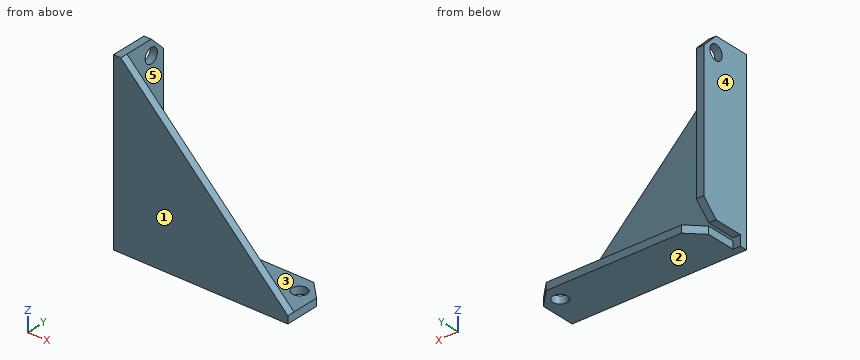
```python
from build123d import *

# Parameters (mm, degrees)
BOSS_EXTRUDE1_DEPTH = 3.175
SKETCH2_W           = 71.842048969
SKETCH2_H           = 3.175
BOSS_EXTRUDE2_DEPTH = 18.923
SKETCH3_W           = 3.175
SKETCH3_H           = 70.598963312
BOSS_EXTRUDE6_DEPTH = 18.923
CUT_EXTRUDE1_DEPTH  = 18.923
CUT_EXTRUDE2_DEPTH  = 18.923
SKETCH7_R           = 3.175
CUT_EXTRUDE3_DEPTH  = 18.923
SKETCH6_R           = 3.175
CUT_EXTRUDE4_DEPTH  = 18.923


with BuildPart() as part:
    # Sketch1 → Boss-Extrude1 (new body)
    with BuildSketch(Plane(origin=(0, 0, 0), x_dir=(1, 0, 0), z_dir=(0, 1, 0))):
        Polygon((-16.345355317, 62.119418011), (58.671693652, 62.119418011), (58.671693652, 58.944418011), (-13.170355317, -12.897630958), (-16.345355317, -12.897630958), align=None)
    extrude(amount=BOSS_EXTRUDE1_DEPTH)

    # Sketch2 → Boss-Extrude2 (add)
    with BuildSketch(Plane(origin=(0, 3.175, 0), x_dir=(1, 0, 0), z_dir=(0, 1, 0))):
        with Locations((22.750669167, 60.531918011)):
            Rectangle(SKETCH2_W, SKETCH2_H)
    extrude(amount=BOSS_EXTRUDE2_DEPTH)

    # Sketch3 → Boss-Extrude6 (add)
    with BuildSketch(Plane(origin=(0, 3.175, 0), x_dir=(1, 0, 0), z_dir=(0, 1, 0))):
        with Locations((-14.757855317, 22.401850698)):
            Rectangle(SKETCH3_W, SKETCH3_H)
    extrude(amount=BOSS_EXTRUDE6_DEPTH)

    # Sketch4 → Cut-Extrude1 (cut)
    with BuildSketch(Plane.ZY.offset(16.345355317)):
        Polygon((6.547630958, 22.098), (12.897630958, 15.748), (12.897630958, 22.098), align=None)
        Polygon((-57.701332354, 22.098), (-57.701332354, 15.748), (-51.351332354, 22.098), align=None)
    extrude(amount=-CUT_EXTRUDE1_DEPTH, mode=Mode.SUBTRACT)

    # Sketch5 → Cut-Extrude2 (cut)
    with BuildSketch(Plane(origin=(0, 0, -62.119418011), x_dir=(-1, 0, 0), z_dir=(0, 0, -1))):
        Polygon((13.170355317, 15.748), (6.820355317, 22.098), (13.170355317, 22.098), align=None)
        Polygon((-58.671693652, 14.834935127), (-51.408628779, 22.098), (-58.671693652, 22.098), align=None)
    extrude(amount=-CUT_EXTRUDE2_DEPTH, mode=Mode.SUBTRACT)

    # Sketch7 → Cut-Extrude3 (cut)
    with BuildSketch(Plane(origin=(-13.170355317, 0, 0), x_dir=(0, 0, -1), z_dir=(1, 0, 0))):
        with Locations((-6.547630958, 15.748)):
            Circle(SKETCH7_R)
    extrude(amount=-CUT_EXTRUDE3_DEPTH, mode=Mode.SUBTRACT)

    # Sketch6 → Cut-Extrude4 (cut)
    with BuildSketch(Plane.XY.offset(-58.944418011)):
        with Locations((51.408628779, 14.834935127)):
            Circle(SKETCH6_R)
    extrude(amount=-CUT_EXTRUDE4_DEPTH, mode=Mode.SUBTRACT)


solid = part.part
```
Could you check a few things on this model? Use its own coordinates, in mm. Face numbers are marked on the shaded views. A direction names the side the tool comes from. Round coordinates to 2 decimals unless told otherwise and drop trailing zeros. Loops run counter-clockwise (first coordinate to the right, second up) from the corner with the lowest first, then second, coordinate; pieces in that order, holes last. Notation, with made-up numbers: M -30,87 L -19,87 A20 cw -19,117 Z; hole C 22.25,-22 d1. An arc over 180 degrees is marked long. Write item = value, one per line.
1. Will these pins go through, and if not, where does the flat tip stop? P1, Ø5, axis at y = 15.75, z = 6.55, coming from the -X side; P2, Ø1, axis at y = 7.5, z = -60.5, coming from the -X side; P3, Ø2.5, axis at x = -14.5, y = 10, coming from the -Z side; P4, Ø10, axis at x = 5.5, y = 12.5, coming from the +Z side.
Results below:
P1 = through
P2 = -13.17
P3 = -57.7
P4 = -58.94
2. I want a section at C-C, the plane x = 14.5. Write out the boundary of the cut face in (y, z) (3 decimals), and give its area (3 significant figures).
Results below:
outline = M 0,-62.119 L 22.098,-62.119 L 22.098,-58.944 L 3.175,-58.944 L 3.175,-14.773 L 0,-14.773 Z
area = 210 mm²
3. I want a section at D-D, the plane z = -30.5. Write out the boundary of the cut face in (x, y) (3 decimals), and give its area (3 significant figures).
Results below:
outline = M -16.345,0 L 30.227,0 L 30.227,3.175 L -13.17,3.175 L -13.17,22.098 L -16.345,22.098 Z
area = 208 mm²
4. Which directions (+Z, -Z, +X, -X, +Y, -Y) give clear straight access to the entire face, cutting with the end or side of a thin tool? Please do the marked faces 3, 4 and 5.
Results below:
face_3 = +Z, +X, -X, +Y
face_4 = +Z, -Z, -X, +Y, -Y
face_5 = +Z, +X, +Y
5. I need wall thicknesses on probe 1 along Z at (x, y) = (53, 20.25); probe 2 along Y at (x, z) = (-12, -15) (3 decimals); probe 3 along X at (y, z) = (4.5, -6). Which ranges of each line are inside material? Lowest first, please.
Results below:
probe_1 = -62.12 to -58.94
probe_2 = 0 to 3.175
probe_3 = -16.35 to -13.17
6. I want a section at A-A, the plane y = 8. Write out the boundary of the cut face in (x, z), and give its area (3 significant figures).
Results below:
outline = M -16.35,-57.7 L -13.17,-57.7 L -13.17,12.9 L -16.35,12.9 Z; M -13.17,-62.12 L 58.67,-62.12 L 58.67,-58.94 L -13.17,-58.94 Z
area = 452 mm²
7. I want a section at B-B, the plane z = 5.5. Write out the boundary of the cut face in (x, y) (3 decimals).
Results below:
outline = M -16.345,0 L -5.773,0 L -5.773,3.175 L -13.17,3.175 L -13.17,12.751 L -16.345,12.751 Z; M -16.345,18.745 L -13.17,18.745 L -13.17,22.098 L -16.345,22.098 Z
8. Thinking about a two-plate mould opening in Y: for the marked faces 1 and 2, which applies, +Y half, -Y half, draft (parallel to the pull), parting line (faces both ways), or undercut?
Results below:
face_1 = -Y half
face_2 = draft
